from build123d import *

# Parameters (mm, degrees)
PAD001_DEPTH = 11.6
PAD_DEPTH    = 13.2
PAD002_DEPTH = 9
PAD003_DEPTH = 9


with BuildPart() as frontal:
    # Sketch001 → Pad001 (new body)
    with BuildSketch(Plane.XZ.offset(-24.2)):
        with BuildLine():
            Line((-24.2, 57.8), (-8.6, 57.8))
            Line((-8.6, 42.8), (-8.6, 57.8))
            ThreePointArc((-8.6, 42.8), (0, 34.2), (8.6, 42.8))
            Line((8.6, 57.8), (8.6, 42.8))
            Line((8.6, 57.8), (24.2, 57.8))
            Line((24.2, 57.8), (24.2, 13.2))
            Line((24.2, 13.2), (-24.2, 13.2))
            Line((-24.2, 13.2), (-24.2, 57.8))
        make_face()
    extrude(amount=PAD001_DEPTH)


with BuildPart() as obj1:
    # Sketch → Pad (new body)
    with BuildSketch(Plane.XY):
        with BuildLine():
            Line((-24.2, 24.2), (24.2, 24.2))
            Line((24.2, 24.2), (24.2, -19.2))
            ThreePointArc((19.2, -24.2), (22.735534, -22.735534), (24.2, -19.2))
            Line((19.2, -24.2), (-19.2, -24.2))
            ThreePointArc((-24.2, -19.2), (-22.735534, -22.735534), (-19.2, -24.2))
            Line((-24.2, -19.2), (-24.2, 24.2))
        make_face()
        with BuildLine():
            Line((7, 4.8), (7, -9.2))
            ThreePointArc((-7, -9.2), (0, -16.2), (7, -9.2))
            Line((-7, -9.2), (-7, 4.8))
            ThreePointArc((7, 4.8), (0, 11.8), (-7, 4.8))
        make_face(mode=Mode.SUBTRACT)
    extrude(amount=PAD_DEPTH)

    # Fusion: union Frontal
    add(frontal.part)


with BuildPart() as escuadra_izquierda:
    # Sketch002 → Pad002 (new body)
    with BuildSketch(Plane.YZ.offset(-24.2)):
        Polygon((-10.2, 13.2), (12.6, 13.2), (12.6, 36), align=None)
    extrude(amount=PAD002_DEPTH)


with BuildPart() as obj2:
    # Sketch003 → Pad003 (new body)
    with BuildSketch(Plane.YZ.offset(24.2)):
        Polygon((-10.2, 13.2), (12.6, 13.2), (12.6, 36), align=None)
    extrude(amount=-PAD003_DEPTH)

    # Fusion001: union Escuadra-izquierda
    add(escuadra_izquierda.part)

    # Fusion002: union obj1
    add(obj1.part)


solid = obj2.part
Verification items for the finished model (mm, model axes). A direction names the side the tool comes from. Coordinates: 2 decimals unless noted, no trailing zeros. Loops run counter-clockwise (first coordinate to the right, second up) from the corner with the lowest first, then second, coordinate; pieces in that order, holes last. Notation, with made-up numbers: (56, 77.5) -> (78, 77.5) arc R20 ccw to (78, 91.5) -> close; hole circle Ø11 at (48, 23). An arc over 180 degrees is marked (long way). Answer as a JSON object with one key per item and string values. Group by question number.
Item 1: Sectioned sample at B-B on x = 0. Record the boundary of the cut face in (y, z).
Item 2: Scan lines: probe 1 along X at (y, z) = (8, 26.5); probe 2 along Y at (x, z) = (-19.5, 44); probe 3 along Z at (x, y) = (-6, 11). Record each from-to range of solid material in increasing order.
Item 3: Sectioned sample at A-A on z = 48. Record the boundary of the cut face in (x, y).
Item 4: Depth check by flat-ended pin: pin 1 (12 mm diameter, centred on x = -4, y = 4, fed in from +Z). Enter the tip coordinate at first touch or a pass-through.
Item 5: Tool access check on faces 1 (the flat face through (6, 12.6, 36)), 2 (the flat face through (-7, -2, 7)), 3 (the flat face through (8.6, 18, 50)). Record the directions out of +Z, -Z, +X, -X, +Y, -Y that give a thin tool (end or side, any length) a straight path to the whole face; none if there is none.
Item 6: Mould release check, pull along X, two halves, no side actions. Record for faces 4 (the cylindrical face through (0.15, 11.8, 6.51)), 5 (the flat face through (-17, 18, 57.8)), 6 (the cylindrical face through (-22.77, -22.7, 6.51)), 7 (the cylindrical face through (-0.15, -16.2, 6.51)): +X half, -X half, draft (parallel to the pull), parting line (faces both ways), or undercut.
Item 7: Sectioned sample at D-D on y = 2. Record the boundary of the cut face in (x, z), plus the area to 3 significant figures.
Item 8: Sectioned sample at C-C on y = 15.5. Record the boundary of the cut face in (x, z), plus the area to 3 significant figures.
Evaluation:
{
 "1": {"outline": "(-24.2, 0) -> (-16.2, 0) -> (-16.2, 13.2) -> (-24.2, 13.2) -> close; (11.8, 0) -> (24.2, 0) -> (24.2, 34.2) -> (12.6, 34.2) -> (12.6, 13.2) -> (11.8, 13.2) -> close"},
 "2": {"probe 1": "x = -24.2 to -15.2, 15.2 to 24.2", "probe 2": "y = 12.6 to 24.2", "probe 3": "z = 0 to 13.2"},
 "3": {"outline": "(-24.2, 12.6) -> (-8.6, 12.6) -> (-8.6, 24.2) -> (-24.2, 24.2) -> close; (8.6, 12.6) -> (24.2, 12.6) -> (24.2, 24.2) -> (8.6, 24.2) -> close"},
 "4": {"pin 1": "stops at z = 13.2"},
 "5": {"face 1": "+Z, -Y", "face 2": "+Z, -Z", "face 3": "+Z, +Y, -Y"},
 "6": {"face 4": "undercut", "face 5": "draft", "face 6": "-X half", "face 7": "undercut"},
 "7": {"outline": "(-24.2, 0) -> (-7, 0) -> (-7, 13.2) -> (-15.2, 13.2) -> (-15.2, 25.4) -> (-24.2, 25.4) -> close; (7, 0) -> (24.2, 0) -> (24.2, 25.4) -> (15.2, 25.4) -> (15.2, 13.2) -> (7, 13.2) -> close", "area": "674 mm²"},
 "8": {"outline": "(-24.2, 0) -> (24.2, 0) -> (24.2, 57.8) -> (8.6, 57.8) -> (8.6, 42.8) arc R8.6 cw to (-8.6, 42.8) -> (-8.6, 57.8) -> (-24.2, 57.8) -> close", "area": "2,420 mm²"}
}
